Autodesk Inventor part; units mm, degrees
ref_plane "YZ Plane" through (0, 0, 0) normal (1, 0, 0) x (0, 1, 0)
ref_plane "XZ Plane" through (0, 0, 0) normal (0, 1, 0) x (-1, 0, 0)
ref_plane "XY Plane" through (0, 0, 0) normal (0, 0, 1) x (1, 0, 0)
sketch "Sketch1" plane through (0, 0, 0) normal (0, 1, 0) x (-1, 0, 0)
  point P0 (0, 0)
sketch "Sketch2" plane through (0, 0, 0) normal (0, 1, 0) x (-1, 0, 0)
  line L0 (0, 0) -> (-30, 0)
  line L1 (-30, 0) -> (-30, -30)
  line L2 (-30, -30) -> (0, -30)
  line L3 (0, -30) -> (0, 0)
  line L4 (0, -30) -> (-30, 0) construction
  line L5 (0, 0) -> (-30, -30) construction
  line L6 (-15, -15) -> (0, -15) construction
  line L7 (-15, -15) -> (-30, -15) construction
  line L8 (-15, -15) -> (-15, -30) construction
  line L9 (-15, -15) -> (-15, 0) construction
  line L10 (-15, -15) -> (-9.25, -15) construction
  line L11 (-15, -17.4158) -> (-15, -15) construction
  line L12 (-15, -15) -> (-15, -20.75) construction
  line L13 (-15, -15) -> (-15, -9.25) construction
  line L14 (-15, -15) -> (-9.25, -15) construction
  line L15 (-15, -15) -> (-20.75, -15) construction
  line L16 (-15, -20.75) -> (-9.25, -15) construction
  line L17 (-9.25, -15) -> (-9.25, -20.75) construction
  line L18 (-9.25, -20.75) -> (-15, -20.75) construction
  line L19 (-15, -20.75) -> (-20.75, -20.75) construction
  line L20 (-20.75, -20.75) -> (-20.75, -15) construction
  line L21 (-9.25, -15) -> (-9.25, -9.25) construction
  line L22 (-15, -9.25) -> (-9.25, -9.25) construction
  line L23 (-15, -9.25) -> (-20.75, -9.25) construction
  line L24 (-20.75, -9.25) -> (-20.75, -15) construction
  line L25 (-15, -9.25) -> (-11, -9.25) construction
  line L26 (-15, -9.25) -> (-19, -9.25) construction
  line L27 (-11, -9.25) -> (-19, -9.25)
  line L28 (-11, -9.25) -> (-11, -3.25)
  line L29 (-11, -3.25) -> (-19, -3.25)
  line L30 (-19, -3.25) -> (-19, -9.25)
  line L31 (-11, -20.75) -> (-19, -20.75)
  line L32 (-19, -20.75) -> (-19, -26.75)
  line L33 (-19, -26.75) -> (-11, -26.75)
  line L34 (-11, -26.75) -> (-11, -20.75)
  line L35 (-9.25, -9.25) -> (-9.25, -10.75)
  line L36 (-9.25, -20.75) -> (-9.25, -18.75)
  line L37 (-9.25, -18.75) -> (-9.25, -19.25)
  line L38 (-9.25, -18.75) -> (-9.25, -10.75)
  line L39 (-9.25, -10.75) -> (-3.25, -10.75)
  line L40 (-3.25, -10.75) -> (-3.25, -18.75)
  line L41 (-3.25, -18.75) -> (-9.25, -18.75)
  line L42 (-9.25, -19.25) -> (-20.75, -19.25) construction
  line L43 (-20.75, -19.25) -> (-20.75, -11.25)
  line L44 (-20.75, -11.25) -> (-26.75, -11.25)
  line L45 (-26.75, -11.25) -> (-26.75, -19.25)
  line L46 (-26.75, -19.25) -> (-20.75, -19.25)
  line L47 (-9.25, -18.75) -> (-11.75, -18.75) construction
  line L48 (-11.75, -18.75) -> (-11.75, -10.75) construction
  line L49 (-11.75, -10.75) -> (-9.25, -10.75) construction
  line L50 (-20.75, -19.25) -> (-18.25, -19.25) construction
  line L51 (-18.25, -19.25) -> (-18.25, -11.25) construction
  line L52 (-18.25, -11.25) -> (-20.75, -11.25) construction
  line L53 (-9.25, -10.75) -> (-9.25, -11.75) construction
  line L54 (-9.25, -11.75) -> (-11.75, -11.75) construction
  line L55 (-20.75, -11.25) -> (-20.75, -11.75) construction
  line L56 (-20.75, -11.75) -> (-18.25, -11.75) construction
  line L57 (-11.75, -18.75) -> (-20.75, -18.75) construction
  line L58 (-18.25, -18.75) -> (-18.25, -11.75) construction
  line L59 (-15, -18.75) -> (-14.25, -18.75) construction
  line L60 (-15, -18.75) -> (-15.75, -18.75) construction
  line L61 (-11.75, -18.75) -> (-11.75, -11.75)
  line L62 (-11.75, -18.75) -> (-14.25, -18.75)
  line L63 (-11.75, -11.75) -> (-14.25, -11.75)
  line L64 (-14.25, -18.75) -> (-14.25, -11.75)
  line L65 (-15.75, -18.75) -> (-18.25, -18.75)
  line L66 (-18.25, -18.75) -> (-18.25, -11.75)
  line L67 (-18.25, -11.75) -> (-15.75, -11.75)
  line L68 (-15.75, -11.75) -> (-15.75, -18.75)
  dimension "d0" = 30
  dimension "d1" = 30
  dimension "d3" = 5.75
  dimension "d4" = 5.75
  dimension "d5" = 5.75
  dimension "d6" = 5.75
  dimension "d7" = 4
  dimension "d8" = 4
  dimension "d9" = 6
  dimension "d10" = 6
  dimension "d11" = 8
  dimension "d12" = 1.5
  dimension "d13" = 2
  dimension "d14" = 0.5
  dimension "d15" = 6
  dimension "d16" = 8
  dimension "d17" = 6
  dimension "d18" = 2.5
  dimension "d19" = 2.5
  dimension "d20" = 1
  dimension "d21" = 0.75
  dimension "d22" = 0.75
extrude "Extrusion1" add sketch "Sketch2" against normal blind 5
extrude "Extrusion2" add sketch "Sketch2" against normal blind 2.5 contours L62 L64 L63 L61 | L65 L66 L67 L68
properties part number "switch_test_v1_3DPrint"
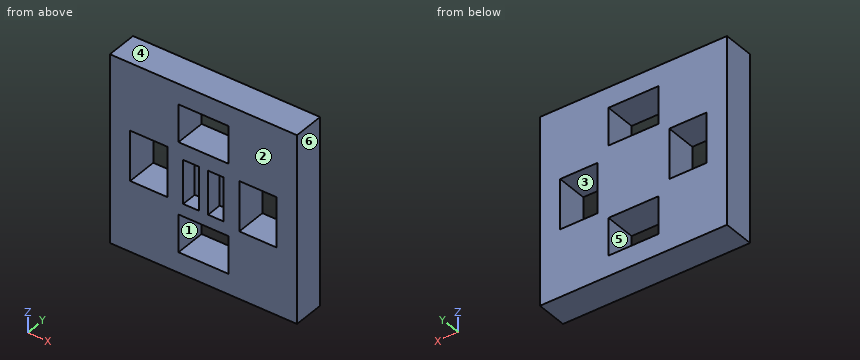
Design review of the part built by this model. Coordinates are the model's own, in mm. Face numbers are marked on the shaded views. A direction names the side the tool comes from. Coordinates: 2 decimals unless noted, no trailing zeros. Order: outer loops, then holes, each group sorted by start corner. A loop starts at its lowest first (then second) coordinate and runs counter-clockwise, first axis right, second up.
1) Wall thickness on line 1 along Z through (x, y) = (18.5, -0.55); line 2 along X through (y, z) = (-2.8, -13); line 3 along Z through (x, y) = (12.5, -3): over which ranges is each line inside the solid? List them lowest first.
2) Mouldability with a two-part tool opening along X and no side actions: class the marked faces 3, 4, 5 and 6 as +X half, -X half, draft (parallel to the pull), parting line (faces both ways), or undercut.
3) Clearance check with a flat-ended pin moving along its axis: pin 1 (0.8 mm diameter, centred on x = 16.5, z = -13.5, fed in from -Y). State where the tip first meets the part, or that it passes through.
4) Take a section at B-B, the plane z = -23. Give the boundary of the cut face in (x, y).
5) Take a section at D-D, the plane x = 13.75. Give the boundary of the cut face in (y, z), and give its area (3 significant figures).
6) For the marked faces 1 and 2, list the 3-axis set-ups (+Z, -Z, +X, -X, +Y, -Y) from which the entire face can be reached by the end or side of a thin tool; tool diameter is ignored.
7) Take a section at C-C, the plane y = -4.5. Give the boundary of the cut face in (x, z), and give its area (3 significant figures).
8) Take a section at A-A, the plane x = 6.5. Give the boundary of the cut face in (y, z).
Returned:
1. line 1: z = -30 to -26.75, -20.75 to -9.25, -3.25 to 0
1. line 2: x = 0 to 3.25, 9.25 to 11.75, 14.25 to 15.75, 18.25 to 20.75, 26.75 to 30
1. line 3: z = -30 to -26.75, -20.75 to -18.75, -11.75 to -9.25, -3.25 to 0
2. face 3: undercut
2. face 4: draft
2. face 5: undercut
2. face 6: +X half
3. pin 1: stops at y = -2.5
4. outline: (0, -5) - (11, -5) - (11, 0) - (0, 0) - close; (19, -5) - (30, -5) - (30, 0) - (19, 0) - close
5. outline: (-5, -30) - (0, -30) - (0, -26.75) - (-5, -26.75) - close; (-5, -20.75) - (0, -20.75) - (0, -9.25) - (-5, -9.25) - (-5, -11.75) - (-2.5, -11.75) - (-2.5, -18.75) - (-5, -18.75) - close; (-5, -3.25) - (0, -3.25) - (0, 0) - (-5, 0) - close
5. area: 72.5 mm2
6. face 1: +Y, -Y
6. face 2: +Z, -Z, +X, -X, -Y
7. outline: (0, -30) - (30, -30) - (30, 0) - (0, 0) - close; hole (3.25, -18.75) - (9.25, -18.75) - (9.25, -10.75) - (3.25, -10.75) - close; hole (11, -26.75) - (19, -26.75) - (19, -20.75) - (11, -20.75) - close; hole (11, -9.25) - (19, -9.25) - (19, -3.25) - (11, -3.25) - close; hole (11.75, -18.75) - (14.25, -18.75) - (14.25, -11.75) - (11.75, -11.75) - close; hole (15.75, -18.75) - (18.25, -18.75) - (18.25, -11.75) - (15.75, -11.75) - close; hole (20.75, -19.25) - (26.75, -19.25) - (26.75, -11.25) - (20.75, -11.25) - close
7. area: 673 mm2
8. outline: (-5, -30) - (0, -30) - (0, -18.75) - (-5, -18.75) - close; (-5, -10.75) - (0, -10.75) - (0, 0) - (-5, 0) - close
